Autodesk Inventor part; units mm, degrees
ref_plane "YZ Plane" through (0, 0, 0) normal (1, 0, 0) x (0, 1, 0)
ref_plane "XZ Plane" through (0, 0, 0) normal (0, 1, 0) x (-1, 0, 0)
ref_plane "XY Plane" through (0, 0, 0) normal (0, 0, 1) x (1, 0, 0)
sketch "Sketch1" plane through (0, 0, 0) normal (0, 0, 1) x (1, 0, 0)
  line L0 (20.6194, 31.3777) -> (22.4899, 31.3777)
  line L1 (22.4899, 31.3777) -> (16.467, 21.1278)
  arc A0 (20.8023, 1.9443) -> (16.467, 21.1278) centre (5.9969, 8.6801) ccw
  line L2 (16.073, 25.8973) -> (18.9256, 30.4411)
  arc A1 (20.6194, 31.3777) -> (18.9256, 30.4411) centre (20.6194, 29.3777) ccw
  line L3 (13.6459, 25.017) -> (15.5204, 25.017)
  line L4 (15.5204, 25.017) -> (16.073, 25.8973)
  arc A2 (17.5545, 3.4219) -> (20.8023, 1.9443) centre (19.1784, 2.6831) ccw
  arc A3 (17.5545, 3.4219) -> (10.3375, 20.6126) centre (5.9969, 8.6801) ccw
  line L5 (9.3399, 23.5753) -> (11.0617, 26.2476)
  line L6 (12.8378, 26.2534) -> (13.6459, 25.017)
  arc A4 (9.3399, 23.5753) -> (10.3375, 20.6126) centre (11.0212, 22.4921) ccw
  arc A5 (12.8378, 26.2534) -> (11.0617, 26.2476) centre (11.9516, 25.6742) ccw
  point P0 (0, 0)
  point P1 (7.8374, 21.2434)
  dimension "d6" = 2
  dimension "d53" = 2
extrude "Extrusion12" add sketch "Sketch1" along normal blind 7
sketch "Sketch14" plane through (0, 0, 7) normal (0, 0, 1) x (1, 0, 0)
  circle A0 centre (11.2711, 22.5911) radius 0.75
  circle A1 centre (18.9401, 28.0713) radius 0.75
  point P0 (0, 0)
  dimension "d56" = 1.5
  dimension "d57" = 1.5
extrude "Extrusion13" cut sketch "Sketch14" against normal through all
sketch "Sketch15" plane through (0, 0, 0) normal (0, 0, -1) x (-1, 0, 0)
  arc A0 (-12.7572, 23.6392) -> (-10.9318, 20.8046) centre (-11.2711, 22.5911) ccw
  circle A1 centre (-18.9401, 28.0713) radius 0.75
  circle A2 centre (-11.2711, 22.5911) radius 0.75
  line L0 (-22.4899, 31.3777) -> (-20.6194, 31.3777)
  line L1 (-16.467, 21.1278) -> (-22.4899, 31.3777)
  arc A3 (-16.467, 21.1278) -> (-20.8023, 1.9443) centre (-5.9969, 8.6801) ccw
  arc A4 (-20.8023, 1.9443) -> (-17.5545, 3.4219) centre (-19.1784, 2.6831) ccw
  arc A5 (-10.3375, 20.6126) -> (-17.5545, 3.4219) centre (-5.9969, 8.6801) ccw
  arc A6 (-10.3375, 20.6126) -> (-9.3399, 23.5753) centre (-11.0212, 22.4921) ccw
  line L2 (-11.0617, 26.2476) -> (-9.3399, 23.5753)
  arc A7 (-11.0617, 26.2476) -> (-12.8378, 26.2534) centre (-11.9516, 25.6742) ccw
  line L3 (-13.6459, 25.017) -> (-12.8378, 26.2534)
  line L4 (-15.5204, 25.017) -> (-13.6459, 25.017)
  line L5 (-18.9256, 30.4411) -> (-15.5204, 25.017)
  arc A8 (-18.9256, 30.4411) -> (-20.6194, 31.3777) centre (-20.6194, 29.3777) ccw
  line L6 (-10.9318, 20.8046) -> (-10.7125, 20.4694)
  arc A9 (-10.3375, 20.6126) -> (-17.5545, 3.4219) centre (-5.9969, 8.6801) ccw
  line L7 (-13.6459, 25.017) -> (-12.7572, 23.6392)
  point P0 (0, 0)
extrude "Extrusion17" cut sketch "Sketch15" against normal blind 2 contours L7 L3 A7 L2 A6 A5 L6 A0
sketch "Sketch18" plane through (0, 0, 7) normal (0, 0, 1) x (1, 0, 0)
  circle A0 centre (18.9401, 28.0713) radius 0.75
  circle A1 centre (11.2711, 22.5911) radius 0.75
  line L0 (22.4899, 31.3777) -> (20.6194, 31.3777)
  arc A2 (20.6194, 31.3777) -> (18.9256, 30.4411) centre (20.6194, 29.3777) ccw
  line L1 (18.9256, 30.4411) -> (15.5204, 25.017)
  line L2 (15.5204, 25.017) -> (13.6459, 25.017)
  line L3 (13.6459, 25.017) -> (12.8378, 26.2534)
  arc A3 (12.8378, 26.2534) -> (11.0617, 26.2476) centre (11.9516, 25.6742) ccw
  line L4 (11.0617, 26.2476) -> (9.3399, 23.5753)
  arc A4 (9.3399, 23.5753) -> (10.3375, 20.6126) centre (11.0212, 22.4921) ccw
  arc A5 (17.5545, 3.4219) -> (10.3375, 20.6126) centre (5.9969, 8.6801) ccw
  arc A6 (17.5545, 3.4219) -> (20.8023, 1.9443) centre (19.1784, 2.6831) ccw
  arc A7 (20.8023, 1.9443) -> (16.467, 21.1278) centre (5.9969, 8.6801) ccw
  line L5 (16.467, 21.1278) -> (22.4899, 31.3777)
  line L6 (16.467, 21.1278) -> (22.4899, 31.3777)
  line L7 (15.5204, 25.017) -> (15.8591, 24.8043)
  line L8 (17.8813, 23.5348) -> (17.5365, 23.7374)
  arc A8 (15.8591, 24.8043) -> (17.5365, 23.7374) centre (16.8393, 24.4933) ccw
  point P0 (0, 0)
  dimension "d75" = 0.4
  dimension "d76" = 0.4
extrude "Extrusion18" cut sketch "Sketch18" against normal blind 2.605 contours L5 L8 A8 L7 L1 A2 L0
sketch "Sketch19" plane through (12.7572, 23.6392, 0) normal (-0.8403389, 0.5420613, 0) x (0, 0, 1)
  line L0 (0, 0) -> (0, 1.6395)
  line L1 (0, 0) -> (2, 0)
  line L2 (2, 0) -> (2, 1.6395)
  line L3 (0, 1.6395) -> (2, 1.6395)
  circle A0 centre (1, 0.8198) radius 0.25
  line L4 (0, 0) -> (2, 0)
  line L5 (2, 1.6395) -> (0, 0)
  line L6 (0, 0) -> (0, 1.6395)
  line L7 (2, 0) -> (0, 1.6395)
  point P0 (0, -26.7801)
  dimension "d79" = 0.5
extrude "Extrusion19" cut sketch "Sketch19" against normal blind 1 contours L5 L7 A0 | A0 L7 L5 | A0 L5 L7 | L7 L5 A0
sketch "Sketch20" plane through (22.4899, 31.3777, 0) normal (0, 0, -1) x (-1, 0, 0)
  line L0 (11.7774, -10.9083) -> (11.5581, -10.5731)
  arc A0 (9.7327, -7.7385) -> (11.5581, -10.5731) centre (11.2188, -8.7866) ccw
  line L1 (9.7327, -7.7385) -> (8.844, -6.3607)
  line L2 (6.9695, -6.3607) -> (8.844, -6.3607)
  line L3 (3.5643, -0.9366) -> (6.9695, -6.3607)
  arc A1 (3.5643, -0.9366) -> (1.8705, 0) centre (1.8705, -2) ccw
  line L4 (0, 0) -> (1.8705, 0)
  line L5 (6.0229, -10.2499) -> (0, 0)
  arc A2 (6.0229, -10.2499) -> (1.6876, -29.4334) centre (16.493, -22.6976) ccw
  arc A3 (1.6876, -29.4334) -> (4.9355, -27.9558) centre (3.3115, -28.6946) ccw
  arc A4 (11.7774, -10.9083) -> (4.9355, -27.9558) centre (16.493, -22.6976) ccw
  circle A5 centre (3.5498, -3.3064) radius 0.75
  line L6 (6.6308, -6.5734) -> (6.9695, -6.3607)
  arc A6 (4.9534, -7.6403) -> (6.6308, -6.5734) centre (5.6506, -6.8844) ccw
  line L7 (4.6086, -7.8429) -> (4.9534, -7.6403)
  point P0 (22.4899, -31.3777)
extrude "Extrusion20" cut sketch "Sketch20" against normal blind 0.475 contours L6 A6 L7 L5 L4 A1 L3
sketch "Sketch22" plane through (20.6194, 31.3777, 4.395) normal (0, 0, 1) x (1, 0, 0)
  circle A0 centre (-1.6793, -3.3064) radius 0.75
  line L0 (0, 0) -> (1.8705, 0)
  arc A1 (0, 0) -> (-1.6939, -0.9366) centre (0, -2) ccw
  line L1 (-5.0991, -6.3607) -> (-1.6939, -0.9366)
  line L2 (-4.7603, -6.5734) -> (-5.0991, -6.3607)
  arc A2 (-4.7603, -6.5734) -> (-3.083, -7.6403) centre (-3.7801, -6.8844) ccw
  line L3 (-2.7381, -7.8429) -> (-3.083, -7.6403)
  line L4 (1.8705, 0) -> (-2.7381, -7.8429)
  line L5 (0, 0) -> (2.0726, 0)
  line L6 (2.0726, 0) -> (2.0726, -0.23)
  arc A3 (2.0726, -0.23) -> (0.5611, -2.2282) centre (5.2352, -4.1929) ccw
  point P0 (-20.6194, -31.3777)
  point P1 (1.2441, -1.066)
  dimension "d99" = 0.23
extrude "Extrusion22" add sketch "Sketch22" against normal up to surface (3.92 mm away) contours L5 L6 A3 L4
fillet "Fillet8" radius 0.1 2 edges at (22.6921, 31.1477, 2.435) (22.6921, 31.3777, 2.435)
sketch "Sketch23" plane through (0, 0, 7) normal (0, 0, 1) x (1, 0, 0)
  line L0 (15.8591, 24.8043) -> (15.5204, 25.017)
  line L1 (15.5204, 25.017) -> (13.6459, 25.017)
  line L2 (13.6459, 25.017) -> (12.8378, 26.2534)
  arc A0 (12.8378, 26.2534) -> (11.0617, 26.2476) centre (11.9516, 25.6742) ccw
  line L3 (11.0617, 26.2476) -> (9.3399, 23.5753)
  arc A1 (9.3399, 23.5753) -> (10.3375, 20.6126) centre (11.0212, 22.4921) ccw
  arc A2 (17.5545, 3.4219) -> (10.3375, 20.6126) centre (5.9969, 8.6801) ccw
  arc A3 (17.5545, 3.4219) -> (20.8023, 1.9443) centre (19.1784, 2.6831) ccw
  arc A4 (20.8023, 1.9443) -> (16.467, 21.1278) centre (5.9969, 8.6801) ccw
  line L4 (16.467, 21.1278) -> (17.8813, 23.5348)
  line L5 (17.8813, 23.5348) -> (17.5365, 23.7374)
  arc A5 (15.8591, 24.8043) -> (17.5365, 23.7374) centre (16.8393, 24.4933) ccw
  circle A6 centre (11.2711, 22.5911) radius 0.75
  point P0 (0, 0)
extrude "Extrusion23" cut sketch "Sketch23" against normal blind 1
properties material "Nickel-Copper Alloy 400"
Geometry: final body of the model. Coordinates: model frame, mm. A direction names the side the tool comes from. Give positions to 0.01 mm unless a question says otherwise; leave off trailing zeros. Write each loop counter-clockwise with the first axis right and the second up, starting at its lowest first coordinate (ties: lowest second). Pieces come first, ordered by that corner, then holes. Notation, with made-up numbers: (21.25, 77.5) - (63.25, 77.5) arc R27 cw to (63.25, 107.5) - close; hole circle Ø1 at (73, 33). An arc over 180 degrees is marked (long way). Return JSON: item names as keys, results as strings. Group by question number.
1) Section D-D on z = 1.55. Return the cut outline in (x, y), plus the area to 3 significant figures.
2) Mould query, pull axis X, two halves, no side actions, for faces 4 (the cylindrical face through (22.2, 30.7, 2.5)), 5 (the flat face through (18, 15, 6)), 6 (the flat face through (15, 25.017, 3)), 7 (the cylindrical face through (11.933, 26.733, 3.972)). Classes: released by +X, released by -X, zero draft, split by the parting line, or undercut.
3) Section A-A on y = 23. Return the cut outline in (x, z), plus the area to 3 significant figures.
4) Section B-B on x = 21.25. Return the cut outline in (y, z) (3 decimals), plus the area to 3 significant figures.
5) First-contact query: P1, Ø3, axis at y = 5.5, z = 2.5, coming from the +X side; P2, Ø1.5, axis at x = 14.5, z = 2.5, coming from the +Y side; P3, Ø3.5, axis at x = 19.5, y = 26, coming from the -Z side (3 decimals); P4, Ø1.4, axis at x = 18.94, y = 28.07, coming from the -Z side. Flat tips, straight axial feed; report the tip coordinate or a pass-through.
6) Set-up query: faces 1 (the flat face through (13.24, 25.64, 3.97)), 2 (the flat face through (22, 31.378, 2)), 3 (the cylindrical face through (16.272, 23.636, 5.209)). Return all of +Z, -Z, +X, -X, +Y, -Y with unobstructed straight access to the full face (end or side cutting, diameter ignored); none if empty.
7) Line query: line 1 (Y direction, x = 17.75, z = 0.9); line 2 (X direction, y = 23, z = 4.1); line 3 (Z direction, x = 13.25, y = 25). Output: solid intervals per line, ascending.
8) Section C-C on z = 4. Return the cut outline in (x, y).
Filled in:
{
 "1": {"outline": "(10.71, 20.47) arc R12.7 cw to (17.55, 3.42) arc R1.78 ccw to (20.8, 1.94) arc R16.27 ccw to (16.47, 21.13) - (21.86, 30.31) arc R5.07 cw to (22.66, 31.12) arc R0.1 ccw to (22.69, 31.2) - (22.69, 31.28) arc R0.1 ccw to (22.59, 31.38) - (20.62, 31.38) arc R2 ccw to (18.93, 30.44) - (16.07, 25.9) - (15.52, 25.02) - (13.65, 25.02) - (12.76, 23.64) arc R1.82 cw to (10.93, 20.8) - close; hole circle Ø1.5 at (18.94, 28.07)", "area": "116 mm^2"},
 "2": {"face 4": "released by +X", "face 5": "zero draft", "face 6": "undercut", "face 7": "undercut"},
 "3": {"outline": "(9.09, 2) - (10.64, 2) - (10.64, 6) - (9.09, 6) - close; (11.9, 2) - (13.04, 2) - (13.04, 0) - (17.57, 0) - (17.57, 6) - (11.9, 6) - close", "area": "37.9 mm^2"},
 "4": {"outline": "(3.031, 0) - (14.329, 0) - (14.329, 6) - (3.031, 6) - close; (29.268, 0.475) - (31.378, 0.475) - (31.378, 4.395) - (29.268, 4.395) - close", "area": "76.1 mm^2"},
 "5": {"P1": "stops at x = 22.18", "P2": "stops at y = 25.02", "P3": "stops at z = 0.475", "P4": "passes through"},
 "6": {"face 1": "+Z, -Z, +Y", "face 2": "+Z, -Z, +X, -X, +Y", "face 3": "+Z"},
 "7": {"line 1": "y = 1.61 to 3.87, 13.49 to 19.92, 23.31 to 28.57", "line 2": "x = 9.09 to 10.64, 11.9 to 17.57", "line 3": "z = 2 to 6"},
 "8": {"outline": "(9.34, 23.58) arc R2 ccw to (10.34, 20.61) arc R12.7 cw to (17.55, 3.42) arc R1.78 ccw to (20.8, 1.94) arc R16.27 ccw to (16.47, 21.13) - (21.86, 30.31) arc R5.07 cw to (22.66, 31.12) arc R0.1 ccw to (22.69, 31.2) - (22.69, 31.28) arc R0.1 ccw to (22.59, 31.38) - (20.62, 31.38) arc R2 ccw to (18.93, 30.44) - (16.07, 25.9) - (15.52, 25.02) - (13.65, 25.02) - (12.84, 26.25) arc R1.06 ccw to (11.06, 26.25) - close; hole circle Ø1.5 at (11.27, 22.59); hole circle Ø1.5 at (18.94, 28.07)"}
}
